```python
from build123d import *

# Parameters (mm, degrees)
SKETCH1_W           = 12.7
SKETCH1_H           = 17.78
SKETCH1_R           = 1.0922
BOSS_EXTRUDE1_DEPTH = 0.635


with BuildPart() as part:
    # Sketch1 → Boss-Extrude1 (new body, symmetric)
    with BuildSketch(Plane.XY):
        Rectangle(SKETCH1_W, SKETCH1_H)
        with Locations((-4.330703088, 6.35)):
            Circle(SKETCH1_R, mode=Mode.SUBTRACT)
        with Locations((-4.330703088, -6.35)):
            Circle(SKETCH1_R, mode=Mode.SUBTRACT)
    extrude(amount=BOSS_EXTRUDE1_DEPTH, both=True)


solid = part.part
```
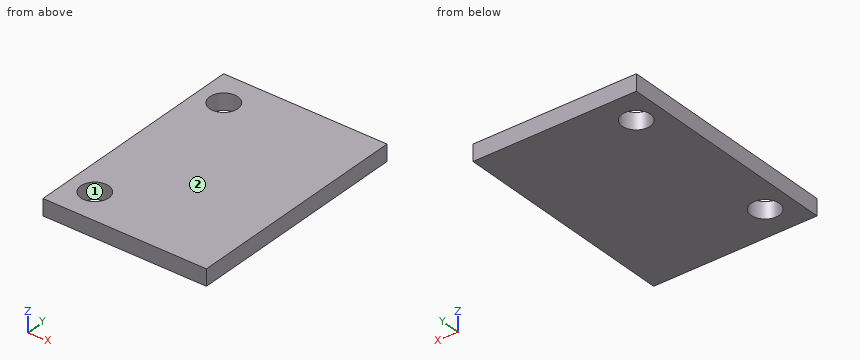
Model file for the job. Use its own axes, mm. Face numbers are marked on the shaded views. Round coordinates to 2 decimals unless told otherwise and drop trailing zeros. Loops run counter-clockwise (first coordinate to the right, second up) from the corner with the lowest first, then second, coordinate; pieces in that order, holes last. Notation, with made-up numbers: M -31.5,41 L 24.5,41 A5 ccw 24.5,45 Z; hole C 40.5,61.25 d7. An arc over 180 degrees is marked long. Put each result on its own line as item: value. Start each with the question number.
Item 1: Cut at B-B (z = 0.2). List the corners of the cut face in (x, y), then the cut area to 3 significant figures.
Item 2: Drill centre lines: line 1 along Y through (x, z) = (-4, 0.25); line 2 along Y through (x, z) = (-3.75, -0.35); line 3 along X through (y, z) = (-5.5, 0.45). Where is each one in solid material? Low to high.
Item 3: Drop a flat-ended pin along its axis: P1, Ø2, axis at x = -4.33, y = -6.35, coming from the +Z side. Give the stop position or say it passes through.
Item 4: Mould opens along X. For the marked faces 1 and 2 say: released by +X, released by -X, zero draft, split by the parting line, or undercut.
Answer block:
1. outline: M -6.35,-8.89 L 6.35,-8.89 L 6.35,8.89 L -6.35,8.89 Z; hole C -4.33,-6.35 d2.18; hole C -4.33,6.35 d2.18
1. area: 218 mm2
2. line 1: -8.89 to -7.39, -5.31 to 5.31, 7.39 to 8.89
2. line 2: -8.89 to -7.28, -5.42 to 5.42, 7.28 to 8.89
2. line 3: -6.35 to -5.02, -3.64 to 6.35
3. P1: through
4. face 1: undercut
4. face 2: zero draft
